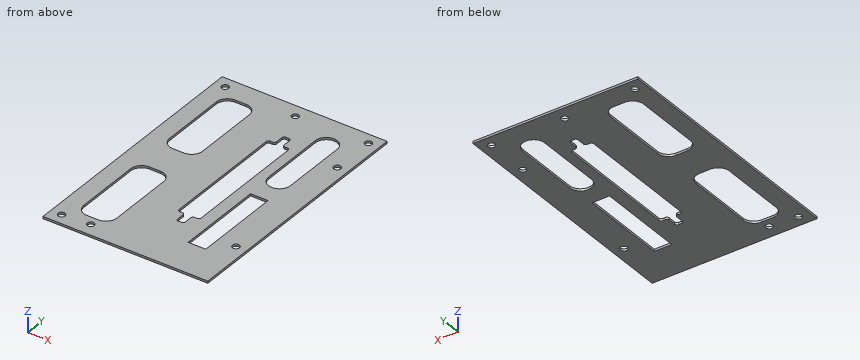
Autodesk Inventor part; units mm, degrees
ref_plane "YZ Plane" through (0, 0, 0) normal (1, 0, 0) x (0, 1, 0)
ref_plane "XZ Plane" through (0, 0, 0) normal (0, 1, 0) x (-1, 0, 0)
ref_plane "XY Plane" through (0, 0, 0) normal (0, 0, 1) x (1, 0, 0)
sketch "Sketch1" plane through (0, 0, 0) normal (0, 0, 1) x (1, 0, 0)
  line L0 (-37.5, 57.5) -> (37.5, 57.5)
  line L1 (37.5, 57.5) -> (37.5, -57.5)
  line L2 (37.5, -57.5) -> (-37.5, -57.5)
  line L3 (-37.5, -57.5) -> (-37.5, 57.5)
  line L4 (-37.5, 57.5) -> (37.5, -57.5) construction
  line L5 (37.5, 57.5) -> (-37.5, -57.5) construction
  line L6 (11, 31.5) -> (11, -24.5)
  line L7 (1, -24.5) -> (1, 31.5)
  line L8 (1, 32.5) -> (11, -25.5) construction
  line L9 (11, 32.5) -> (1, -25.5) construction
  line L10 (5.25, 38) -> (6.75, 38)
  line L11 (7.75, 37) -> (7.75, 33.5)
  line L12 (4.25, 33.5) -> (4.25, 37)
  line L13 (4.25, 38) -> (7.75, 32.5) construction
  line L14 (7.75, 38) -> (4.25, 32.5) construction
  line L15 (5.25, -31) -> (6.75, -31)
  line L16 (7.75, -30) -> (7.75, -26.5)
  line L17 (4.25, -26.5) -> (4.25, -30)
  line L18 (4.25, -31) -> (7.75, -25.5) construction
  line L19 (7.75, -31) -> (4.25, -25.5) construction
  circle A0 centre (-32.6, 52.5) radius 1.6
  line L20 (0, 0) -> (0, 3.4669)
  line L21 (0, 0) -> (3.1568, 0)
  circle A1 centre (32.6, 52.5) radius 1.6
  circle A2 centre (-32.6, -52.5) radius 1.6
  circle A3 centre (-20, -51.5) radius 1.6
  circle A4 centre (32.6, -32.5) radius 1.6
  circle A5 centre (32.6, 32.5) radius 1.6
  circle A6 centre (0, 51.5) radius 1.6
  line L22 (16.5, -0.5) -> (24.5, -0.5)
  line L23 (24.5, -0.5) -> (24.5, -40.5)
  line L24 (24.5, -40.5) -> (16.5, -40.5)
  line L25 (16.5, -40.5) -> (16.5, -0.5)
  line L26 (16.5, -0.5) -> (24.5, -40.5) construction
  line L27 (24.5, -0.5) -> (16.5, -40.5) construction
  line L28 (-24.5, 47.5) -> (-19.5, 47.5)
  line L29 (-14.5, 42.5) -> (-14.5, 12.5)
  line L30 (-19.5, 7.5) -> (-24.5, 7.5)
  line L31 (-29.5, 12.5) -> (-29.5, 42.5)
  line L32 (-29.5, 47.5) -> (-14.5, 7.5) construction
  line L33 (-14.5, 47.5) -> (-29.5, 7.5) construction
  arc A7 (-24.5, 47.5) -> (-29.5, 42.5) centre (-24.5, 42.5) ccw
  arc A8 (-14.5, 42.5) -> (-19.5, 47.5) centre (-19.5, 42.5) ccw
  arc A9 (-19.5, 7.5) -> (-14.5, 12.5) centre (-19.5, 12.5) ccw
  arc A10 (-29.5, 12.5) -> (-24.5, 7.5) centre (-24.5, 12.5) ccw
  line L34 (-24.5, -47.5) -> (-19.5, -47.5)
  line L35 (-14.5, -42.5) -> (-14.5, -12.5)
  line L36 (-19.5, -7.5) -> (-24.5, -7.5)
  line L37 (-29.5, -12.5) -> (-29.5, -42.5)
  line L38 (-29.5, -47.5) -> (-14.5, -7.5) construction
  line L39 (-14.5, -47.5) -> (-29.5, -7.5) construction
  arc A11 (-29.5, -42.5) -> (-24.5, -47.5) centre (-24.5, -42.5) ccw
  arc A12 (-19.5, -47.5) -> (-14.5, -42.5) centre (-19.5, -42.5) ccw
  arc A13 (-14.5, -12.5) -> (-19.5, -7.5) centre (-19.5, -12.5) ccw
  arc A14 (-24.5, -7.5) -> (-29.5, -12.5) centre (-24.5, -12.5) ccw
  line L40 (20.5, 47.5) -> (20.5, 47.5)
  line L41 (25.5, 42.5) -> (25.5, 12.5)
  line L42 (20.5, 7.5) -> (20.5, 7.5)
  line L43 (15.5, 12.5) -> (15.5, 42.5)
  line L44 (15.5, 47.5) -> (25.5, 7.5) construction
  line L45 (25.5, 47.5) -> (15.5, 7.5) construction
  arc A15 (20.5, 47.5) -> (15.5, 42.5) centre (20.5, 42.5) ccw
  arc A16 (25.5, 42.5) -> (20.5, 47.5) centre (20.5, 42.5) ccw
  arc A17 (20.5, 7.5) -> (25.5, 12.5) centre (20.5, 12.5) ccw
  arc A18 (15.5, 12.5) -> (20.5, 7.5) centre (20.5, 12.5) ccw
  arc A19 (5.25, 38) -> (4.25, 37) centre (5.25, 37) ccw
  arc A20 (7.75, 37) -> (6.75, 38) centre (6.75, 37) ccw
  arc A21 (4.25, -30) -> (5.25, -31) centre (5.25, -30) ccw
  arc A22 (6.75, -31) -> (7.75, -30) centre (6.75, -30) ccw
  line L46 (10, -25.5) -> (8.75, -25.5)
  line L47 (3.25, -25.5) -> (2, -25.5)
  line L48 (2, 32.5) -> (3.25, 32.5)
  line L49 (8.75, 32.5) -> (10, 32.5)
  arc A23 (2, 32.5) -> (1, 31.5) centre (2, 31.5) ccw
  arc A24 (3.25, 32.5) -> (4.25, 33.5) centre (3.25, 33.5) ccw
  arc A25 (7.75, 33.5) -> (8.75, 32.5) centre (8.75, 33.5) ccw
  arc A26 (11, 31.5) -> (10, 32.5) centre (10, 31.5) ccw
  arc A27 (10, -25.5) -> (11, -24.5) centre (10, -24.5) ccw
  arc A28 (8.75, -25.5) -> (7.75, -26.5) centre (8.75, -26.5) ccw
  arc A29 (4.25, -26.5) -> (3.25, -25.5) centre (3.25, -26.5) ccw
  arc A30 (1, -24.5) -> (2, -25.5) centre (2, -24.5) ccw
  point P0 (6, 3.5)
  point P1 (6, 35.25)
  point P2 (6, -28.25)
  point P3 (20.5, -20.5)
  point P4 (-22, 27.5)
  point P5 (-22, -27.5)
  point P6 (20.5, 27.5)
  point P7 (0, -57.5)
  point P8 (0, 57.5)
  dimension "d0" = 75
  dimension "d1" = 115
  dimension "d2" = 3.5
  dimension "d3" = 5.5
  dimension "d4" = 10
  dimension "d5" = 58
  dimension "d6" = 26.5
  dimension "d9" = 3.2
  dimension "d10" = 5
  dimension "d11" = 4.9
  dimension "d14" = 3.2
  dimension "d15" = 6
  dimension "d16" = 3.2
  dimension "d18" = 4.9
  dimension "d19" = 25
  dimension "d20" = 8
  dimension "d21" = 40
  dimension "d23" = 13
  dimension "d24" = 17
  dimension "d25" = 15
  dimension "d26" = 40
  dimension "d27" = 5
  dimension "d28" = 10
  dimension "d29" = 8
  dimension "d30" = 40
  dimension "d31" = 10
  dimension "d32" = 12
  dimension "d33" = 10
  dimension "d34" = 5
  dimension "d36" = 20
  dimension "d37" = 6
  dimension "d38" = 0
  dimension "d39" = 3.2
  dimension "d40" = 1
  dimension "d41" = 25
  dimension "d42" = 1
extrude "Plate1" add sketch "Sketch1" along normal blind 1
equation "\"d8\" = 厚度"
equation "\"折彎半徑\" = 厚度"
equation "\"折彎離隙寬度\" = 厚度"
equation "\"折彎離隙深度\" = 0.5 * 厚度"
equation "\"轉角離隙大小\" = 4 * 厚度"
equation "\"最小剩餘\" = 2 * 厚度"
equation "\"轉移半徑\" = 折彎半徑"
equation "\"Jacobi半徑大小\" = 折彎半徑"
equation "\"間隙大小\" = 厚度"
properties part number "PCB_board_box_back" material "Aluminum"
Geometry check sheet. Reference: the model listing, model coordinates, mm. Give positions to 0.01 mm unless a question says otherwise; leave off trailing zeros. Write each loop counter-clockwise with the first axis right and the second up, starting at its lowest first coordinate (ties: lowest second). Pieces come first, ordered by that corner, then holes.
1) Section check A-A, the plane y = -23. Record the boundary of the cut face in (x, z).
2) Material ranges on L1, parallel to X at y = 36, z = 0.65; L2, parallel to X at y = 12.5, z = 0.55; L3, parallel to X at y = -3.5, z = 0.6, recorded low to high.
3) Gauge pin test, flat end, axial feed: pin 1 (5 mm diameter, centred on x = 32.6, y = 32.5, fed in from -Z). Record the tip position at first contact, or that the pin passes through.
4) Section check D-D, the plane x = 32.6. Record the boundary of the cut face in (y, z), and give its area (3 significant figures).
5) Section check B-B, the plane x = -32.6. Record the boundary of the cut face in (y, z), and give its area (3 significant figures).
6) Section check C-C, the plane y = -45.5. Record the boundary of the cut face in (x, z).
Computed:
1. outline: (-37.5, 0) - (-29.5, 0) - (-29.5, 1) - (-37.5, 1) - close; (-14.5, 0) - (1, 0) - (1, 1) - (-14.5, 1) - close; (11, 0) - (16.5, 0) - (16.5, 1) - (11, 1) - close; (24.5, 0) - (37.5, 0) - (37.5, 1) - (24.5, 1) - close
2. L1: x = -37.5 to -29.5, -14.5 to 4.25, 7.75 to 15.5, 25.5 to 37.5
2. L2: x = -37.5 to -29.5, -14.5 to 1, 11 to 15.5, 25.5 to 37.5
2. L3: x = -37.5 to 1, 11 to 16.5, 24.5 to 37.5
3. pin 1: stops at z = 0
4. outline: (-57.5, 0) - (-34.1, 0) - (-34.1, 1) - (-57.5, 1) - close; (-30.9, 0) - (30.9, 0) - (30.9, 1) - (-30.9, 1) - close; (34.1, 0) - (50.9, 0) - (50.9, 1) - (34.1, 1) - close; (54.1, 0) - (57.5, 0) - (57.5, 1) - (54.1, 1) - close
4. area: 105 mm2
5. outline: (-57.5, 0) - (-54.1, 0) - (-54.1, 1) - (-57.5, 1) - close; (-50.9, 0) - (50.9, 0) - (50.9, 1) - (-50.9, 1) - close; (54.1, 0) - (57.5, 0) - (57.5, 1) - (54.1, 1) - close
5. area: 109 mm2
6. outline: (-37.5, 0) - (-28.5, 0) - (-28.5, 1) - (-37.5, 1) - close; (-15.5, 0) - (37.5, 0) - (37.5, 1) - (-15.5, 1) - close
